Check sheet for the modelled part. Datum: model origin and axes. Units: mm. Face numbers are marked on the shaded views. A direction names the side the tool comes from. Round coordinates to 2 decimals unless told otherwise and drop trailing zeros. Order: outer loops, then holes, each group sorted by start corner. A loop starts at its lowest first (then second) coordinate and runs counter-clockwise, first axis right, second up.
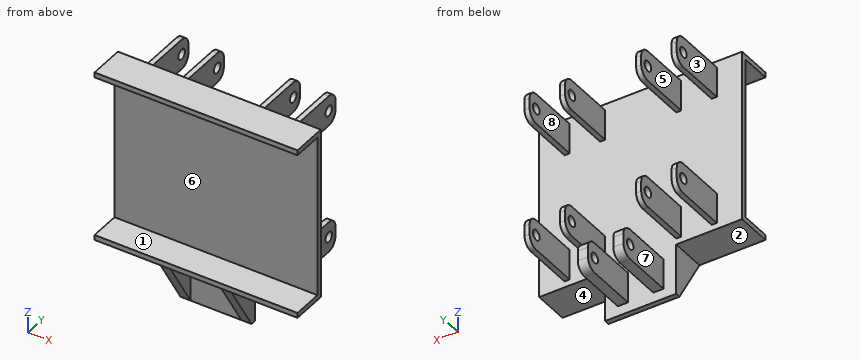
```python
from build123d import *

# Parameters (mm, degrees)
SKETCH2_W              = 200
SKETCH2_H              = 160
BOSS_EXTRUDE1_DEPTH    = 5
SKETCH3_W              = 5
SKETCH3_H              = 30
BOSS_EXTRUDE2_DEPTH    = 60
CUT_EXTRUDE1_REACH     = 171.853
SKETCH4_R              = 5
FILLET1_R              = 10
LPATTERN1_COUNT        = 2
LPATTERN1_PITCH        = 110
LPATTERN1_COUNT_DIR2   = 2
LPATTERN1_PITCH_DIR2   = 127.98756405
FILLET1_OF_LPATTERN1_R = 10
SKETCH6_W              = 200
SKETCH6_H              = 35
BOSS_EXTRUDE3_DEPTH    = 5
SKETCH7_W              = 70
SKETCH7_H              = 5
BOSS_EXTRUDE8_DEPTH    = 50
SKETCH9_W              = 10
SKETCH9_H              = 30
BOSS_EXTRUDE9_DEPTH    = 60
FILLET2_R              = 10
CUT_EXTRUDE2_REACH     = 195.536
SKETCH11_R             = 5
RIB4_REACH             = 203.68
SKETCH14_WALL_W        = 463.67039955
SKETCH14_WALL_H        = 10


with BuildPart() as part:
    # Sketch2 → Boss-Extrude1 (new body)
    with BuildSketch(Plane(origin=(0, 0, 0), x_dir=(1, 0, 0), z_dir=(0, 1, 0))):
        Rectangle(SKETCH2_W, SKETCH2_H)
    extrude(amount=BOSS_EXTRUDE1_DEPTH)

    # Sketch3 → Boss-Extrude2 (add)
    with BuildSketch(Plane(origin=(0, 5, 0), x_dir=(1, 0, 0), z_dir=(0, 1, 0))):
        with Locations((-72.5, 63.98756405)):
            Rectangle(SKETCH3_W, SKETCH3_H)
        with Locations((-37.5, 63.98756405)):
            Rectangle(SKETCH3_W, SKETCH3_H)
    boss_extrude2 = extrude(amount=BOSS_EXTRUDE2_DEPTH)

    # Cut-Extrude1: up to this face of the body (flat: up to its plane)
    cut_extrude1_end = Plane(part.part.faces().sort_by_distance((-75, 35, -63.98756405))[0])
    # Sketch4 → Cut-Extrude1 (cut, up to the picked face)
    with BuildSketch(Plane(origin=(-35, 0, 0), x_dir=(0, 0, -1), z_dir=(1, 0, 0)), mode=Mode.PRIVATE) as cut_extrude1_sk1:
        with Locations((63.98756405, 55)):
            Circle(SKETCH4_R)
    cut_extrude1_tool1 = split(extrude(cut_extrude1_sk1.sketch, amount=-CUT_EXTRUDE1_REACH, mode=Mode.PRIVATE), bisect_by=cut_extrude1_end, keep=Keep.BOTH, mode=Mode.PRIVATE)
    cut_extrude1 = cut_extrude1_tool1.solids().sort_by(Axis((-35, 55, -63.987564), (-1, 0, 0)))[0]
    add(cut_extrude1, mode=Mode.SUBTRACT)

    # Fillet1
    fillet1_edges = [part.edges().sort_by_distance(p)[0] for p in [
        (-72.5, 65, -78.98756405),
        (-72.5, 65, -48.98756405),
        (-37.5, 65, -78.98756405),
        (-37.5, 65, -48.98756405),
    ]]
    fillet(fillet1_edges, radius=FILLET1_R)

    # LPattern1: Boss-Extrude2, Cut-Extrude1 2 × 2
    with Locations(*[(i * LPATTERN1_PITCH, 0, j * LPATTERN1_PITCH_DIR2) for i in range(LPATTERN1_COUNT) for j in range(LPATTERN1_COUNT_DIR2) if (i, j) != (0, 0)]):
        add(boss_extrude2)
        add(cut_extrude1, mode=Mode.SUBTRACT)

    # Fillet1 of LPattern1
    fillet1_of_lpattern1_edges = [part.edges().sort_by_distance(p)[0] for p in [
        (-72.5, 65, 49),
        (-72.5, 65, 79),
        (-37.5, 65, 49),
        (-37.5, 65, 79),
        (37.5, 65, -78.98756405),
        (37.5, 65, -48.98756405),
        (72.5, 65, -78.98756405),
        (72.5, 65, -48.98756405),
        (37.5, 65, 49),
        (37.5, 65, 79),
        (72.5, 65, 49),
        (72.5, 65, 79),
    ]]
    fillet(fillet1_of_lpattern1_edges, radius=FILLET1_OF_LPATTERN1_R)

    # Sketch6 → Boss-Extrude3 (add)
    with BuildSketch(Plane(origin=(0, 0, -80), x_dir=(-1, 0, 0), z_dir=(0, 0, -1))):
        with Locations((0, -12.5)):
            Rectangle(SKETCH6_W, SKETCH6_H)
    boss_extrude3 = extrude(amount=BOSS_EXTRUDE3_DEPTH)

    # Mirror8: Boss-Extrude3 across plane
    add(boss_extrude3.mirror(Plane.XY))

    # Sketch7 → Boss-Extrude8 (add)
    with BuildSketch(Plane(origin=(0, 0, -85), x_dir=(-1, 0, 0), z_dir=(0, 0, -1))):
        with Locations((0, 2.5)):
            Rectangle(SKETCH7_W, SKETCH7_H)
    extrude(amount=BOSS_EXTRUDE8_DEPTH)

    # Sketch9 → Boss-Extrude9 (add)
    with BuildSketch(Plane(origin=(0, 5, 0), x_dir=(1, 0, 0), z_dir=(0, 1, 0))):
        with Locations((-17.5, 110)):
            Rectangle(SKETCH9_W, SKETCH9_H)
        with Locations((17.5, 110)):
            Rectangle(SKETCH9_W, SKETCH9_H)
    extrude(amount=BOSS_EXTRUDE9_DEPTH)

    # Fillet2
    fillet2_edges = [part.edges().sort_by_distance(p)[0] for p in [
        (-17.5, 65, -95),
        (-17.5, 65, -125),
        (17.5, 65, -95),
        (17.5, 65, -125),
    ]]
    fillet(fillet2_edges, radius=FILLET2_R)

    # Cut-Extrude2: up to this face of the body (flat: up to its plane)
    cut_extrude2_end = Plane(part.part.faces().sort_by_distance((-22.5, 34.321749192, -110))[0])
    # Sketch11 → Cut-Extrude2 (cut, up to the picked face)
    with BuildSketch(Plane(origin=(22.5, 0, 0), x_dir=(0, 0, -1), z_dir=(1, 0, 0)), mode=Mode.PRIVATE) as cut_extrude2_sk1:
        with Locations((110, 55)):
            Circle(SKETCH11_R)
    cut_extrude2_tool1 = split(extrude(cut_extrude2_sk1.sketch, amount=-CUT_EXTRUDE2_REACH, mode=Mode.PRIVATE), bisect_by=cut_extrude2_end, keep=Keep.BOTH, mode=Mode.PRIVATE)
    add(cut_extrude2_tool1.solids().sort_by(Axis((22.5, 55, -110), (-1, 0, 0)))[0], mode=Mode.SUBTRACT)

    # Sketch14 wall → Rib4 (add, up to next)
    with BuildSketch(Plane(origin=(35, -15, -110), x_dir=(0, -0.514495755428, 0.857492925713), z_dir=(0, -0.857492925713, -0.514495755428)), mode=Mode.PRIVATE) as rib4_sk1:
        with Locations((0, 5)):
            Rectangle(SKETCH14_WALL_W, SKETCH14_WALL_H)
    rib4_tool1 = extrude(rib4_sk1.sketch, amount=-RIB4_REACH, mode=Mode.PRIVATE) - part.part
    rib4 = rib4_tool1.solids().sort_by_distance((35, -15, -110))[0]
    add(rib4)

    # Mirror1: Rib4 across plane
    add(rib4.mirror(Plane(origin=(0, 0, 0), x_dir=(0, 0, 1), z_dir=(1, 0, 0))))


solid = part.part
```
Item 1: Scan lines: line 1 along X through (y, z) = (16, -65); line 2 along Y through (x, z) = (36.95, 64); line 3 along Y through (x, z) = (17.5, 34). Record each from-to range of solid material in increasing order.
Answer:
line 1: x = -75 to -70, -40 to -35, 35 to 40, 70 to 75
line 2: y = 0 to 50, 60 to 65
line 3: y = 0 to 5
Item 2: Release check for a two-part mould opening along X. For the marked faces 6, 7 and 8 record: released by +X, released by -X, zero draft, split by the parting line, or undercut.
Answer:
face 6: zero draft
face 7: released by -X
face 8: undercut
Item 3: Access from +Z, -Z, +X, -X, +Y, -Y to the whole of each face (thin tool, end or side, straight path). Record for the marked faces 1, 2, 3, 4 and 5.
Answer:
face 1: +X, -X, -Y
face 2: -Z, -X, +Y, -Y
face 3: +Z, -Z, -X, +Y
face 4: -Z, +X, +Y, -Y
face 5: +Z, -Z, +Y
Item 4: Sectioned sample at A-A (y = -6). Record the cut outline in (x, z).
Answer:
outline: (-100, -85) - (-35, -85) - (-35, -125) - (-25, -125) - (-25, -85) - (25, -85) - (25, -125) - (35, -125) - (35, -85) - (100, -85) - (100, -80) - (-100, -80) - close; (-100, 80) - (100, 80) - (100, 85) - (-100, 85) - close
Item 5: Sectioned sample at B-B (x = 37.5). Record the cut outline in (y, z).
Answer:
outline: (-30, -85) - (5, -85) - (5, -78.99) - (55, -78.99) arc R10 ccw to (65, -68.99) - (65, -58.99) arc R10 ccw to (55, -48.99) - (5, -48.99) - (5, 49) - (55, 49) arc R10 ccw to (65, 59) - (65, 69) arc R10 ccw to (55, 79) - (5, 79) - (5, 85) - (-30, 85) - (-30, 80) - (0, 80) - (0, -80) - (-30, -80) - close; hole circle Ø10 at (55, -63.99); hole circle Ø10 at (55, 64)
Item 6: Go/stop test with flat-tipped pins: P1, Ø3, axis at x = -19.5, y = 29.5, coming from the -Z side; P2, Ø11.5, axis at y = 55, z = -63.99, coming from the -X side; P3, Ø8, axis at x = -67.5, z = -58, coming from the -Y side. Record where each tip stops, or that it passes through.
Answer:
P1: stops at z = -125
P2: stops at x = -75
P3: stops at y = 0
Item 7: Sectioned sample at C-C (z = -110). Record the cut outline in (x, y).
Answer:
outline: (-35, -15) - (-25, -15) - (-25, 0) - (25, 0) - (25, -15) - (35, -15) - (35, 5) - (22.5, 5) - (22.5, 50) - (12.5, 50) - (12.5, 5) - (-12.5, 5) - (-12.5, 50) - (-22.5, 50) - (-22.5, 5) - (-35, 5) - close; (-22.5, 60) - (-12.5, 60) - (-12.5, 65) - (-22.5, 65) - close; (12.5, 60) - (22.5, 60) - (22.5, 65) - (12.5, 65) - close
Item 8: Sectioned sample at D-D (x = -9.5). Record the cut outline in (y, z).
Answer:
outline: (-30, -85) - (0, -85) - (0, -135) - (5, -135) - (5, 85) - (-30, 85) - (-30, 80) - (0, 80) - (0, -80) - (-30, -80) - close
